```python
from build123d import *

# Parameters (mm, degrees)
SKETCH1_W           = 120.5
SKETCH1_H           = 120.5
SKETCH1_W_2         = 110.5
SKETCH1_H_2         = 110.5
BOSS_EXTRUDE1_DEPTH = 23
SKETCH2_W           = 120.5
SKETCH2_H           = 120.5
BOSS_EXTRUDE2_DEPTH = 3
SKETCH3_W           = 17.5
SKETCH3_H           = 100.5
CUT_EXTRUDE1_DEPTH  = 47
CUT_EXTRUDE2_DEPTH  = 47
CUT_EXTRUDE3_DEPTH  = 47
SKETCH7_W           = 120.5
SKETCH7_H           = 10
SKETCH7_R           = 2.5
BOSS_EXTRUDE3_DEPTH = 3


with BuildPart() as part:
    # Sketch1 → Boss-Extrude1 (new body)
    with BuildSketch(Plane.XY):
        Rectangle(SKETCH1_W, SKETCH1_H)
        Rectangle(SKETCH1_W_2, SKETCH1_H_2, mode=Mode.SUBTRACT)
    extrude(amount=BOSS_EXTRUDE1_DEPTH)

    # Sketch2 → Boss-Extrude2 (add)
    with BuildSketch(Plane(origin=(0, 0, 0), x_dir=(-1, 0, 0), z_dir=(0, 0, -1))):
        Rectangle(SKETCH2_W, SKETCH2_H)
    extrude(amount=BOSS_EXTRUDE2_DEPTH)

    # Sketch3 → Cut-Extrude1 (cut)
    with BuildSketch(Plane(origin=(-55.25, 0, 0), x_dir=(0, 0, -1), z_dir=(1, 0, 0))):
        with Locations((-14.25, 0)):
            Rectangle(SKETCH3_W, SKETCH3_H)
    extrude(amount=-CUT_EXTRUDE1_DEPTH, mode=Mode.SUBTRACT)

    # Sketch5 → Cut-Extrude2 (cut)
    with BuildSketch(Plane.XZ.offset(-55.25)):
        Polygon((-37.75, 23), (-37.75, 14), (-21.25, 14), (-21.25, 0), (21.25, 0), (21.25, 14), (15.25, 14), (15.25, 23), align=None)
    extrude(amount=-CUT_EXTRUDE2_DEPTH, mode=Mode.SUBTRACT)

    # Sketch6 → Cut-Extrude3 (cut)
    with BuildSketch(Plane.ZY.offset(-55.25)):
        Polygon((23, 45.25), (5.5, 45.25), (5.5, 27.75), (13, 27.75), (13, -55.25), (23, -55.25), align=None)
    extrude(amount=-CUT_EXTRUDE3_DEPTH, mode=Mode.SUBTRACT)

    # Sketch7 → Boss-Extrude3 (add)
    # profile 1 of 2: a face of its own
    with BuildSketch(Plane(origin=(0, 0, -3), x_dir=(-1, 0, 0), z_dir=(0, 0, -1))):
        with Locations((0, 65.25)):
            Rectangle(SKETCH7_W, SKETCH7_H)
        with Locations((-52.75, 65.25)):
            Circle(SKETCH7_R, mode=Mode.SUBTRACT)
        with Locations((-42.75, 65.25)):
            Circle(SKETCH7_R, mode=Mode.SUBTRACT)
        with Locations((52.75, 65.25)):
            Circle(SKETCH7_R, mode=Mode.SUBTRACT)
        with Locations((42.75, 65.25)):
            Circle(SKETCH7_R, mode=Mode.SUBTRACT)
    # profile 2 of 2: a face of its own
    with BuildSketch(Plane(origin=(0, 0, -3), x_dir=(-1, 0, 0), z_dir=(0, 0, -1))):
        with Locations((0, -65.25)):
            Rectangle(SKETCH7_W, SKETCH7_H)
        with Locations((-52.75, -65.25)):
            Circle(SKETCH7_R, mode=Mode.SUBTRACT)
        with Locations((-42.75, -65.25)):
            Circle(SKETCH7_R, mode=Mode.SUBTRACT)
        with Locations((42.75, -65.25)):
            Circle(SKETCH7_R, mode=Mode.SUBTRACT)
        with Locations((52.75, -65.25)):
            Circle(SKETCH7_R, mode=Mode.SUBTRACT)
    extrude(amount=-BOSS_EXTRUDE3_DEPTH)


solid = part.part
```
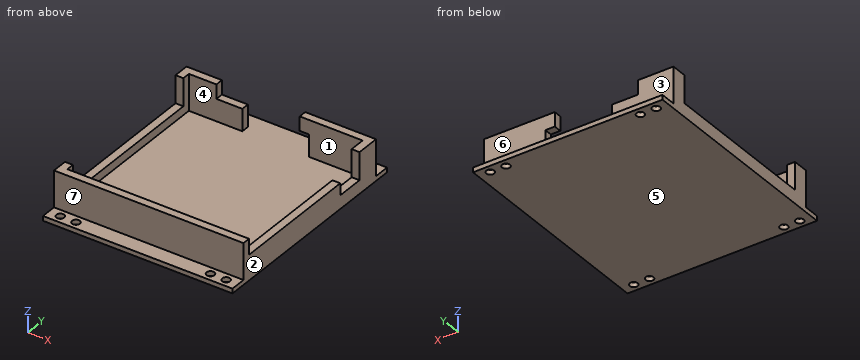
Here's how the part is built. I have some questions about the finished solid (model axes, mm). Face numbers are marked on the shaded views. A direction names the side the tool comes from. Give positions to 0.01 mm unless a question says otherwise; leave off trailing zeros. Loops run counter-clockwise (first coordinate to the right, second up) from the corner with the lowest first, then second, coordinate; pieces in that order, holes last. Notation, with made-up numbers: M 71,61.25 L 114,61.25 A18 ccw 114,69.25 Z; hole C 78,4.5 d8. An arc over 180 degrees is marked long. Use one line per item in the form item = value. Start each with the question number.
Q1. Which directions (+Z, -Z, +X, -X, +Y, -Y) give clear straight access to the entire face, cutting with the end or side of a thin tool? Please do the marked faces 5, 6 and 7.
Q2. Thinking about a two-plate mould opening in X: for the marked faces 1, 2, 3 and 4, which applies, +X half, -X half, draft (parallel to the pull), parting line (faces both ways), or undercut?
Q3. I need wall thicknesses on line 1 along Y through (x, z) = (42.75, -0.7); line 2 along Y through (x, z) = (32.5, 8.5); line 3 along Z through (x, y) = (-49.5, -25). Which ranges of each line are inside material? Lowest first, please.
Q4. If we section it at D-D (x = -5): Write out the boundary of the cut face in (y, z), then the cut area to 4 significant figures.
Q5. If we section it at C-C (x = 42.75): Write out the boundary of the cut face in (y, z), then the cut area to 4 significant figures.
Q6. If we section it at B-B (y = 52): Write out the boundary of the cut face in (x, z).
Q7. Will these pins go through, and if not, where does the flat tip stop? pin 1 Ø2.5 at (x, y) = (58, 36.5) entering from +Z; pin 2 Ø11.5 at (x, z) = (31.5, 10) entering from -Y; pin 3 Ø6 at (y, z) = (27, 17) entering from +X; pin 4 Ø5.5 at (x, z) = (-59, 16) entering from +Y.
Q8. If we section it at A-A (z = 18.5): Write out the boundary of the cut face in (x, y), then the cut area to 3 significant figures.
Taken from the geometry:
q1.face_5 = -Z, +X, -X, +Y, -Y
q1.face_6 = +Z, +X, -X, +Y
q1.face_7 = +Z, +X, -X, -Y
q2.face_1 = undercut
q2.face_2 = +X half
q2.face_3 = draft
q2.face_4 = undercut
q3.line_1 = -70.25 to -67.75, -62.75 to 62.75, 67.75 to 70.25
q3.line_2 = -60.25 to -55.25, 55.25 to 60.25
q3.line_3 = -3 to 0
q4.outline = M -70.25,-3 L 70.25,-3 L 70.25,0 L -55.25,0 L -55.25,23 L -60.25,23 L -60.25,0 L -70.25,0 Z
q4.area = 536.5 mm^2
q5.outline = M -70.25,-3 L -67.75,-3 L -67.75,0 L -70.25,0 Z; M -62.75,-3 L 62.75,-3 L 62.75,0 L 60.25,0 L 60.25,23 L 55.25,23 L 55.25,0 L -55.25,0 L -55.25,23 L -60.25,23 L -60.25,0 L -62.75,0 Z; M 67.75,-3 L 70.25,-3 L 70.25,0 L 67.75,0 Z
q5.area = 621.5 mm^2
q6.outline = M -60.25,-3 L 60.25,-3 L 60.25,23 L 55.25,23 L 55.25,0 L -55.25,0 L -55.25,23 L -60.25,23 Z
q7.pin_1 = 5.5
q7.pin_2 = -60.25
q7.pin_3 = through
q7.pin_4 = 60.25
q8.outline = M -60.25,-60.25 L 60.25,-60.25 L 60.25,-55.25 L -55.25,-55.25 L -55.25,-50.25 L -60.25,-50.25 Z; M -60.25,50.25 L -55.25,50.25 L -55.25,55.25 L -37.75,55.25 L -37.75,60.25 L -60.25,60.25 Z; M 15.25,55.25 L 55.25,55.25 L 55.25,45.25 L 60.25,45.25 L 60.25,60.25 L 15.25,60.25 Z
q8.area = 1,040 mm^2
